Input: part model. Units: mm. Frame: model coordinates. A direction names the side the tool comes from. Give positions to 0.01 mm unless a question says otherwise; leave off trailing zeros. Order: outer loops, then holes, each group sorted by start corner. A loop starts at its lowest first (then second) coordinate and runs counter-clockwise, first axis right, second up. Notation, with made-up numbers: (72.5, -2) - (109.5, -2) arc R32 ccw to (109.5, 34) - close; hole circle Ø6 at (51, 40). An arc over 180 degrees is marked (long way). Use a Markdown table: item, result.
from build123d import *

# Parameters (mm, degrees)
ESBO_O1_R                = 1.6
ESBO_O1_R_2              = 0.7499985
RESSALTO_EXTRUS_O1_DEPTH = 3
FILETE1_R                = 1
FILETE2_R                = 6
FILETE3_R                = 8
FILETE4_R                = 8


with BuildPart() as part:
    # Esboço1 → Ressalto-extrusão1 (new body)
    with BuildSketch(Plane.XY):
        Polygon((78.115114297, 18.654012354), (78.115114297, 12.154012354), (43.115114297, -2.345987646), (18.715114297, -2.345987646), (-16.284885703, 12.154012354), (-16.284885703, 18.654012354), (-9.784885703, 18.654012354), (-1.784885703, 18.654012354), (18.702505635, 14.138058789), (43.102505635, 14.138058789), (63.615114297, 18.654012354), (71.615114297, 18.654012354), align=None)
        with Locations((74.865114297, 15.154012354)):
            Circle(ESBO_O1_R, mode=Mode.SUBTRACT)
        with Locations((-13.034885703, 15.154012354)):
            Circle(ESBO_O1_R, mode=Mode.SUBTRACT)
        with Locations((21.915114517, -0.245988346)):
            Circle(ESBO_O1_R_2, mode=Mode.SUBTRACT)
        with Locations((39.915114077, -0.245988346)):
            Circle(ESBO_O1_R_2, mode=Mode.SUBTRACT)
        with Locations((64.415113337, 17.154012414)):
            Circle(ESBO_O1_R_2, mode=Mode.SUBTRACT)
        with Locations((-2.584884743, 17.154012414)):
            Circle(ESBO_O1_R_2, mode=Mode.SUBTRACT)
        Polygon((19.709836187, 2.654012354), (-4.773656813, 12.79717374), (18.308653057, 9.138058789), (43.496014169, 9.138058789), (66.607059688, 12.798488799), (42.120392408, 2.654012354), align=None, mode=Mode.SUBTRACT)
    extrude(amount=RESSALTO_EXTRUS_O1_DEPTH)

    # Filete1
    filete1_edges = [part.edges().sort_by_distance(p)[0] for p in [
        (66.607059688, 12.798488799, 1.5),
        (-4.773656813, 12.79717374, 1.5),
    ]]
    fillet(filete1_edges, radius=FILETE1_R)

    # Filete2
    filete2_edges = [part.edges().sort_by_distance(p)[0] for p in [
        (19.709836187, 2.654012354, 1.5),
        (42.120392408, 2.654012354, 1.5),
        (43.496014169, 9.138058789, 1.5),
        (18.308653057, 9.138058789, 1.5),
    ]]
    fillet(filete2_edges, radius=FILETE2_R)

    # Filete3
    filete3_edges = [part.edges().sort_by_distance(p)[0] for p in [
        (43.115114297, -2.345987646, 1.5),
        (18.715114297, -2.345987646, 1.5),
        (18.702505635, 14.138058789, 1.5),
        (43.102505635, 14.138058789, 1.5),
    ]]
    fillet(filete3_edges, radius=FILETE3_R)

    # Filete4
    filete4_edges = [part.edges().sort_by_distance(p)[0] for p in [
        (-1.784885703, 18.654012354, 1.5),
        (63.615114297, 18.654012354, 1.5),
    ]]
    fillet(filete4_edges, radius=FILETE4_R)


solid = part.part
1. Mould query, pull axis X, two halves, no side actions, for faces 1 (the face through (78.115, 15, 1)), 2 (the face through (51.122, 6.383, 1.479)), 3 (the face through (31, -2.346, 1)). Classes: pulls with the +X half, pulls with the -X half, needs draft (parallel to the pull), parting line crosses it, or undercut.
Response:
| item | result |
|---|---|
| face 1 | pulls with the +X half |
| face 2 | undercut |
| face 3 | needs draft |
2. Set-up query: faces 4 (the face through (43.106, -2.188, 1.521)), 5 (the face through (19.72, 2.77, 1.52)), 6 (the face through (31, 14.138, 1)). Return all of +Z, -Z, +X, -X, +Y, -Y with unobstructed straight access to the full face (end or side cutting, diameter ignored); none if empty.
Response:
| item | result |
|---|---|
| face 4 | +Z, -Z, +X, -Y |
| face 5 | +Z, -Z |
| face 6 | +Z, -Z, +Y |
3. Section query B-B (z = 1.7). State how many separate pieces and enclosed holes the cut face has, then the cut area to 3 significant figures.
Response:
| item | result |
|---|---|
| separate pieces | 1 |
| enclosed holes | 7 |
| area | 964 mm^2 |
4. Material intervals for line 1 along Y through (x, z) = (20.5, 1.8); line 2 along Y through (x, z) = (10, 1); line 3 along X through (y, z) = (6, 2.3), sorted ascending.
Response:
| item | result |
|---|---|
| line 1 | y = -2.35 to 2.67, 9.14 to 14.14 |
| line 2 | y = 1.26 to 6.68, 10.46 to 16.06 |
| line 3 | x = -1.43 to 11.63, 50.2 to 63.26 |
5. Section query A-A (x = 37.5). Return loops of the section in (y, z), then the cut area to 3 significant figures.
Response:
| item | result |
|---|---|
| outline | (-2.35, 0) - (2.65, 0) - (2.65, 3) - (-2.35, 3) - close; (9.14, 0) - (14.14, 0) - (14.14, 3) - (9.14, 3) - close |
| area | 30.0 mm^2 |
6. Section query C-C (y = 6.75). Return loops of the section in (x, z), then the cut area to 3 significant figures.
Response:
| item | result |
|---|---|
| outline | (-3.24, 0) - (9.82, 0) - (9.82, 3) - (-3.24, 3) - close; (52.01, 0) - (65.07, 0) - (65.07, 3) - (52.01, 3) - close |
| area | 78.4 mm^2 |
7. Pin query (flat end, axial travel): pin 1 (1 mm diameter, centred on x = 1, z = 1, fed in from +Y). Return the tip coordinate at first contact, or that it passes through.
Response:
| item | result |
|---|---|
| pin 1 | stops at y = 18.15 |
8. Section query D-D (x = 71). Return loops of the section in (y, z), then the cut area to 3 significant figures.
Response:
| item | result |
|---|---|
| outline | (9.21, 0) - (18.65, 0) - (18.65, 3) - (9.21, 3) - close |
| area | 28.3 mm^2 |
